Autodesk Inventor part; units mm, degrees
ref_plane "Work Plane1" through (-11.7757, -19.1185, 0) normal (0, 0, 1) x (1, 0, 0)
ref_plane "YZ Plane" through (0, 0, 0) normal (1, 0, 0) x (0, 1, 0)
ref_plane "XZ Plane" through (0, 0, 0) normal (0, 1, 0) x (-1, 0, 0)
sketch "Sketch1" plane through (0, 0, 0) normal (0, 0, 1) x (1, 0, 0)
  line L0 (5.7396, -16.8109) -> (-2.4232, -6.7282)
  line L1 (-2.4232, -6.7282) -> (-8.3008, 0.7051)
  arc A0 (10.2494, 10.2845) -> (-8.3008, 0.7051) centre (0.0414, 7.3014) ccw
  arc A1 (2.7914, -3.3149) -> (10.2494, 10.2845) centre (0.2126, 6.944) ccw
  line L2 (2.7914, -3.3149) -> (5.9881, -7.541)
  arc A2 (6.711, -5.8652) -> (5.9881, -7.541) centre (19.909, -12.5525) ccw
  line L3 (6.711, -5.8652) -> (5.8177, -4.6842)
  arc A3 (5.8177, -4.6842) -> (11.7757, 8.697) centre (-6.2296, 8.697) ccw
  arc A4 (11.7757, 8.697) -> (2.54, 18.8513) centre (0.0414, 7.3014) ccw
  line L4 (-9.2281, -0.0281) -> (-2.54, -8.4863)
  line L5 (2.9614, -15.4438) -> (6.6502, -19.1185)
  arc A5 (5.7396, -16.8109) -> (6.6502, -19.1185) centre (19.909, -12.5525) ccw
  arc A6 (6.711, -5.8652) -> (6.6502, -19.1185) centre (19.909, -12.5525) ccw
  circle A7 centre (0.0414, 7.3014) radius 4.3509
  circle A8 centre (0, 21.4919) radius 1.27
  line L6 (2.54, 18.8513) -> (2.54, 21.4919)
  arc A9 (2.54, 21.4919) -> (-2.54, 21.4919) centre (0, 21.4919) ccw
  line L7 (-2.54, 21.4919) -> (-2.54, 18.8331)
  arc A10 (-2.54, 18.8331) -> (-9.2281, -0.0281) centre (0.0414, 7.3014) ccw
  circle A11 centre (0, -15.0639) radius 1.27
  line L8 (-2.54, -8.4863) -> (-2.54, -15.0639)
  arc A12 (-2.54, -15.0639) -> (2.54, -15.0639) centre (0, -15.0639) ccw
  line L9 (2.54, -15.0639) -> (2.54, -14.9108)
  line L10 (2.54, -14.9108) -> (2.9614, -15.4438)
  point P0 (0, 0)
extrude "Extrusion1" add sketch "Sketch1" along normal blind 1.7 contours A5 L5 L10 L9 A12 L8 L4 A10 L7 A9 L6 A4 A3 L3 A2 L2 A1 A0 L1 L0 | L0 L1 A0 A1 L2 A6 | A8 | A11
sketch "Sketch2" plane through (0, 0, 1.7) normal (0, 0, 1) x (1, 0, 0)
  circle A0 centre (0, 21.4919) radius 1.524
  circle A1 centre (0, -15.0639) radius 1.524
  line L0 (2.54, 17.6957) -> (-2.54, 17.6957)
  line L1 (-2.54, 17.6957) -> (-2.54, 21.4919)
  line L2 (2.54, 17.6957) -> (2.54, 21.4919)
  arc A2 (2.54, 21.4919) -> (-2.54, 21.4919) centre (0, 21.4919) ccw
  arc A3 (-2.54, -15.0639) -> (2.54, -15.0639) centre (0, -15.0639) ccw
  line L3 (-2.54, -15.0639) -> (-2.54, -7.1979)
  line L4 (-2.54, -7.1979) -> (2.54, -12.2319)
  line L5 (2.54, -12.2319) -> (2.54, -15.0639)
  point P0 (0, 0)
  dimension "d2" = 3.048
  dimension "d3" = 3.048
  dimension "d4" = 2.54
  dimension "d5" = 2.54
ref_plane "Work Plane1" through (-11.7757, -19.1185, 0) normal (0, 0, 1) x (1, 0, 0)
sketch "Sketch3" plane through (0, 0, 1.7) normal (0, 0, 1) x (1, 0, 0)
  line L0 (-7.5086, 0.6681) -> (-7.5086, 13.9346)
  arc A0 (7.5914, 13.9346) -> (-7.5086, 13.9346) centre (0.0414, 7.3014) ccw
  arc A1 (-7.5086, 0.6681) -> (7.5914, 0.6681) centre (0.0414, 7.3014) ccw
  line L1 (7.5914, 13.9346) -> (7.5914, 0.6681)
  arc A2 (-7.7626, 0.5731) -> (7.8454, 0.5731) centre (0.0414, 7.3014) ccw
  line L2 (-7.7626, 0.5731) -> (-7.7626, 14.0297)
  arc A3 (7.8454, 14.0297) -> (-7.7626, 14.0297) centre (0.0414, 7.3014) ccw
  line L3 (7.8454, 14.0297) -> (7.8454, 0.5731)
  arc A4 (-9.2757, 0.0326) -> (9.3585, 0.0326) centre (0.0414, 7.3014) ccw
  line L4 (-9.2757, 0.0326) -> (-9.2757, 14.5702)
  arc A5 (9.3585, 14.5702) -> (-9.2757, 14.5702) centre (0.0414, 7.3014) ccw
  line L5 (9.3585, 14.5702) -> (9.3585, 0.0326)
  line L6 (-9.2281, -0.0281) -> (-2.54, -8.4863)
  line L7 (2.9614, -15.4438) -> (6.6502, -19.1185)
  arc A6 (6.711, -5.8652) -> (6.6502, -19.1185) centre (19.909, -12.5525) ccw
  line L8 (6.711, -5.8652) -> (5.8177, -4.6842)
  arc A7 (5.8177, -4.6842) -> (11.7757, 8.697) centre (-6.2296, 8.697) ccw
  arc A8 (11.7757, 8.697) -> (2.54, 18.8513) centre (0.0414, 7.3014) ccw
  circle A9 centre (0.0414, 7.3014) radius 4.3509
  arc A10 (11.7757, 8.697) -> (2.54, 18.8513) centre (0.0414, 7.3014) ccw
  line L9 (2.54, 18.8513) -> (2.54, 21.4919)
  arc A11 (2.54, 21.4919) -> (-2.54, 21.4919) centre (0, 21.4919) ccw
  line L10 (-2.54, 21.4919) -> (-2.54, 18.8331)
  arc A12 (-2.54, 18.8331) -> (-9.2281, -0.0281) centre (0.0414, 7.3014) ccw
  line L11 (-2.54, -8.4863) -> (-2.54, -15.0639)
  arc A13 (-2.54, -15.0639) -> (2.54, -15.0639) centre (0, -15.0639) ccw
  line L12 (2.54, -15.0639) -> (2.54, -14.9108)
  line L13 (2.54, -14.9108) -> (2.9614, -15.4438)
  point P0 (0, 0)
  dimension "d8" = 0.254
extrude "Extrusion3" add sketch "Sketch3" along normal blind 12.7 contours L4 A5 L5 A4
extrude "Extrusion4" cut sketch "Sketch2" against normal blind 12.7 contours A0 | A1
sketch "Sketch4" plane through (0, 0, 0) normal (0, 1, 0) x (-1, 0, 0)
  line L0 (9.2757, 14.4) -> (-9.3585, 14.4)
  line L1 (9.2757, 1.7) -> (9.2757, 14.4)
  line L2 (-9.3585, 1.7) -> (-9.3585, 14.4)
  line L3 (2.54, 1.7) -> (-2.54, 1.7)
  line L4 (2.54, 1.7) -> (-2.54, 1.7)
  line L5 (2.54, 1.7) -> (2.54, 8.05)
  line L6 (-2.54, 1.7) -> (-2.54, 8.05)
  arc A0 (2.54, 8.05) -> (-2.54, 8.05) centre (0, 8.05) ccw
  point P0 (0, 0)
  point P1 (-9.3585, 8.05)
extrude "Extrusion5" add sketch "Sketch4" against normal blind 9.525
sketch "Sketch5" plane through (0, 0, 14.4) normal (0, 0, 1) x (1, 0, 0)
  line L0 (-7.7626, 0.5731) -> (-7.7626, 14.0297)
  arc A0 (7.8454, 14.0297) -> (-7.7626, 14.0297) centre (0.0414, 7.3014) ccw
  line L1 (7.8454, 14.0297) -> (7.8454, 0.5731)
  arc A1 (-7.7626, 0.5731) -> (7.8454, 0.5731) centre (0.0414, 7.3014) ccw
  line L2 (9.3585, 0.0326) -> (9.3585, 14.5702)
  arc A2 (9.3585, 14.5702) -> (-9.2757, 14.5702) centre (0.0414, 7.3014) ccw
  line L3 (-9.2757, 14.5702) -> (-9.2757, 0.0326)
  arc A3 (-9.2757, 0.0326) -> (9.3585, 0.0326) centre (0.0414, 7.3014) ccw
  point P0 (0, 0)
extrude "Extrusion6" cut sketch "Sketch5" against normal up to surface (12.7 mm away) contours L0 A0 L1 A1
sketch "Sketch6" plane through (0, -9.525, 0) normal (0, -1, 0) x (1, 0, 0)
  circle A0 centre (0, 8.05) radius 1.016
  arc A1 (2.54, 8.05) -> (-2.54, 8.05) centre (0, 8.05) ccw
  point P0 (0, 0)
  dimension "d17" = 2.032
extrude "Extrusion7" cut sketch "Sketch6" against normal blind 12.7
properties part number "Motor Holder"
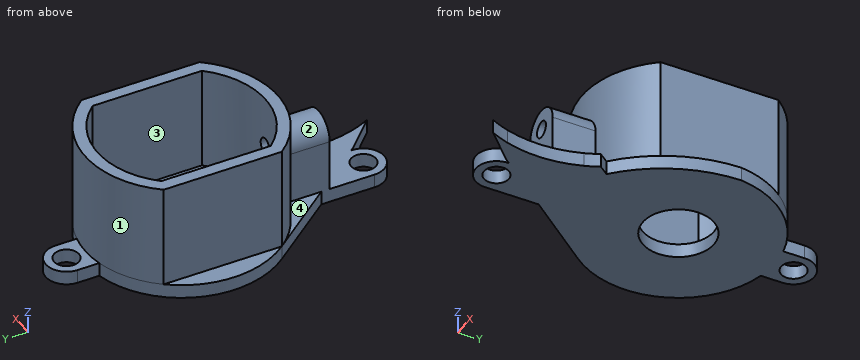
Work out the finished part from the listing and answer in its coordinate system (mm). Face numbers are marked on the shaded views. A direction names the side the tool comes from. Round coordinates to 2 decimals unless told otherwise and drop trailing zeros. Write each loop counter-clockwise with the first axis right and the second up, starting at its lowest first coordinate (ties: lowest second). Pieces come first, ordered by that corner, then holes. Notation, with made-up numbers: (22, 80.5) - (75, 80.5) arc R11 cw to (75, 90.5) - close; hole circle Ø8 at (-17, 59.25). An arc over 180 degrees is marked (long way). Answer in a Markdown table with one row per item. Add a question column.
1. Given pin 1 (4 mm diameter, centred on y = 5, z = 7.5, fed in from +X); pin 2 (6.5 mm diameter, centred on y = -12, z = 4.5, fed in from -X); pin 3 (7 mm diameter, centred on x = 3.5, y = -8, fed in from +Z); pin 4 (2.5 mm diameter, centred on x = 0, y = 21.49, fed in from -Z), each flat-ended and moving along its own axis, determine where each tip first touches the part or whether it passes through.
2. A cutting plane is placed at B-B, the plane x = 0. Count the separate pieces of the cut face and the enclosed holes in it, and give its area (3 significant figures).
3. Find the intervals of material crossed by line 1 along Y through (x, z) = (0, 0.8); line 2 along X through (y, z) = (7, 2.25); line 3 along X through (y, z) = (-6, 8.05), in increasing order. Write a range as from..to.
4. A cutting plane is placed at A-A, the plane z = 12. Determine the outline of the cut face in (x, y).
5. For the marked faces 1, 2, 3 and 4, determine the directions among +Z, -Z, +X, -X, +Y, -Y from which every point of the face is accessible in a straight line to the end or side of a thin tool.
6. A cutting plane is placed at C-C, the plane y = -1. Determine the outline of the cut face in (x, z), and give its area (3 significant figures).
7. A cutting plane is placed at D-D, the plane x = 8.75. Determine the outline of the cut face in (y, z), and give its area (3 significant figures).
Worked out:
| question | item | result |
|---|---|---|
| 1 | pin 1 | x = 9.36 |
| 1 | pin 2 | x = -2.54 |
| 1 | pin 3 | z = 10.59 |
| 1 | pin 4 | through |
| 2 | separate pieces | 5 |
| 2 | enclosed holes | 0 |
| 2 | area | 115 mm^2 |
| 3 | line 1 | -17.6..-16.59, -13.54..2.95, 11.65..19.97, 23.02..24.03 |
| 3 | line 2 | -9.28..-7.76, 7.85..9.36 |
| 3 | line 3 | -2.54..-1.02, 1.02..2.54 |
| 4 | outline | (-9.28, 0.03) arc R11.82 ccw to (9.36, 0.03) - (9.36, 14.57) arc R11.82 ccw to (-9.28, 14.57) - close; hole (-7.76, 0.57) arc R10.3 ccw to (7.85, 0.57) - (7.85, 14.03) arc R10.3 ccw to (-7.76, 14.03) - close |
| 5 | face 1 | +Z, +Y |
| 5 | face 2 | +Z, -Y |
| 5 | face 3 | +Z |
| 5 | face 4 | +Z, -X, -Y |
| 6 | outline | (-8.46, 0) - (8.94, 0) - (8.94, 1.7) - (8.45, 1.7) - (8.45, 14.4) - (6.15, 14.4) - (6.15, 1.7) - (-6.06, 1.7) - (-6.06, 14.4) - (-8.37, 14.4) - (-8.37, 1.7) - (-8.46, 1.7) - close |
| 6 | area | 88.2 mm^2 |
| 7 | outline | (-1.29, 0) - (15.29, 0) - (15.29, 14.4) - (-0.69, 14.4) - (-0.69, 1.7) - (-1.29, 1.7) - close |
| 7 | area | 231 mm^2 |
